Verification items for the finished model (mm, model axes). Give positions to 0.01 mm unless a question says otherwise; leave off trailing zeros. Order: outer loops, then holes, each group sorted by start corner. A loop starts at its lowest first (then second) coordinate and runs counter-clockwise, first axis right, second up.
from build123d import *

# Parameters (mm, degrees)
F1_DEPTH = 25.4


with BuildPart() as f1:
    # F0 (on Right) → F1 (new body)
    with BuildSketch(Plane.YZ):
        with BuildLine():
            Line((46.839244, 48.341449), (-54.760756, 48.341449))
            Line((-54.760756, 48.341449), (-86.152115, -69.798089))
            Line((-86.152115, -69.798089), (-36.191094, -69.798089))
            ThreePointArc((-36.191094, -69.798089), (0.258513, -33.348482), (36.70812, -69.798089))
            Line((36.70812, -69.798089), (86.669141, -69.798089))
            Line((86.669141, -69.798089), (46.839244, 48.341449))
        make_face()
    extrude(amount=F1_DEPTH)


solid = f1.part
(1) Release check for a two-part mould opening along Y. For faces 1 (the cylindrical face through (12.522, -0.543, -33.357)), 2 (the flat face through (12.522, 67.033, -11.555)), 3 (the flat face through (12.522, -70.237, -9.901)), 4 (the flat face through (0, -1, -10)) record: pulls with the +Y half, pulls with the -Y half, needs draft (parallel to the pull), parting line crosses it, or undercut.
Solved:
face 1: undercut
face 2: pulls with the +Y half
face 3: pulls with the -Y half
face 4: needs draft
(2) Section check A-A, the plane z = -38.5. Enter the section's corners in (x, y).
Solved:
outline: (0, -77.84) - (25.4, -77.84) - (25.4, -18.42) - (0, -18.42) - close; (0, 18.94) - (25.4, 18.94) - (25.4, 76.12) - (0, 76.12) - close
(3) Go/stop test with flat-tipped pins: pin 1 (2 mm diameter, centred on x = 17.5, z = -52.5, fed in from -Y); pin 2 (2 mm diameter, centred on x = 22, y = -25.5, fed in from -Z); pin 3 (1 mm diameter, centred on x = 11.5, y = 3, fed in from -Z). Record where each tip stops, or that it passes through.
Solved:
pin 1: stops at y = -81.82
pin 2: stops at z = -45.05
pin 3: stops at z = -33.49
(4) Section check B-B, the plane x = 9. Enter the section's corners in (y, z), then the cut area to 3 significant figures.
Solved:
outline: (-86.15, -69.8) - (-36.19, -69.8) arc R36.45 cw to (36.71, -69.8) - (86.67, -69.8) - (46.84, 48.34) - (-54.76, 48.34) - close
area: 14,100 mm2
(5) Section check D-D, the plane y = -29. Enter the section's corners in (x, z), then the cut area to 3 significant figures.
Solved:
outline: (0, -48.06) - (25.4, -48.06) - (25.4, 48.34) - (0, 48.34) - close
area: 2,450 mm2
(6) Scan lines: line 1 (Y direction, x = 9.5, z = -62); line 2 (Y direction, x = 24, z = -45); line 3 (Z direction, x = 24, y = -5.5). Record each from-to range of solid material in increasing order.
Solved:
line 1: y = -84.08 to -35.35, 35.86 to 84.04
line 2: y = -79.56 to -26.46, 26.97 to 78.31
line 3: z = -33.81 to 48.34
(7) Section check C-C, the plane z = -59.5. Enter the section's corners in (x, y), then the cut area to 3 significant figures.
Solved:
outline: (0, -83.42) - (25.4, -83.42) - (25.4, -34.71) - (0, -34.71) - close; (0, 35.22) - (25.4, 35.22) - (25.4, 83.2) - (0, 83.2) - close
area: 2,460 mm2
